Design review of the part shown in the three views and the two pictorial views. Dimensions are in mm from the part's minimum x, y and z. Coordinates: 2 decimals unless noted, no trailing zeros. Loops run counter-clockwise (first coordinate to the right, second up) from the corner with the lowest first, then second, coordinate; pieces in that order, holes last. Notation, with made-up numbers: M 18,13 L 66,13 A30 ccw 66,46 Z; hole C 37.5,-9.5 d10. An arc over 180 degrees is marked long. Use one line per item in the form item = value.
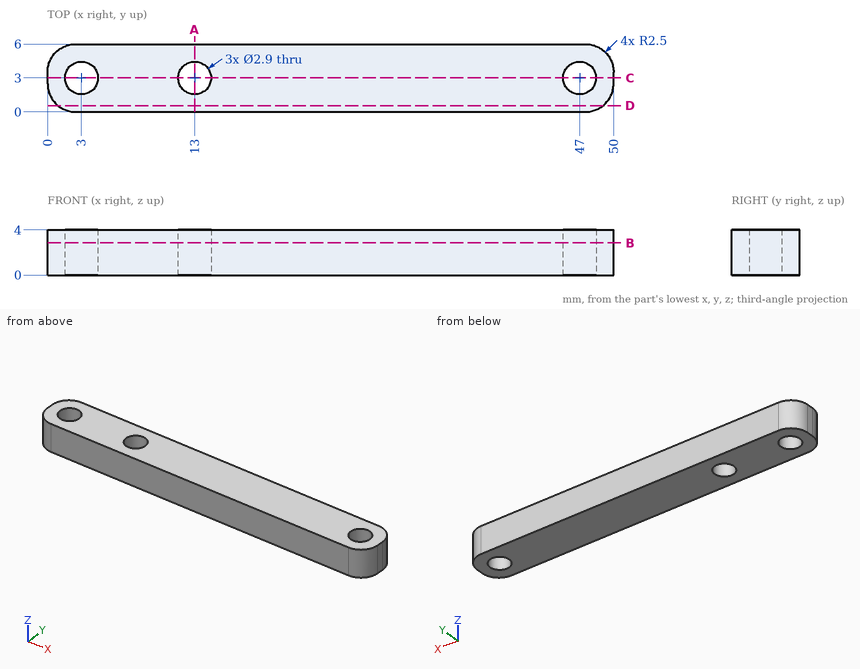
1. Add section D-D (y = 0.55). State the section outline as (x, z) points, then the cut area to 3 significant figures.
Response values:
outline = M 0.94,0 L 49.06,0 L 49.06,4 L 0.94,4 Z
area = 193 mm^2
2. Wall thickness on line 1 along Y through (x, z) = (3, 1.6); line 2 along X through (y, z) = (1.9, 1.3); line 3 along X through (y, z) = (2.2, 2.55): over which ranges is each line inside the solid? List them lowest first. Write a range as from..to.
Response values:
line_1 = 0..1.55, 4.45..6
line_2 = 0.07..2.06, 3.94..12.06, 13.94..46.06, 47.94..49.93
line_3 = 0.02..1.79, 4.21..11.79, 14.21..45.79, 48.21..49.98
3. Insertion check: P1, Ø1, axis at y = 1, z = 2, coming from the +X side. The pin has a flat end and moves straight along its axis. Give the tip position at first contact, or say it passes through.
Response values:
P1 = 49.79
4. Add section B-B (z = 2.85). State the section outline as (x, y) points, then the cut area to 3 significant figures.
Response values:
outline = M 0,2.5 A2.5 ccw 2.5,0 L 47.5,0 A2.5 ccw 50,2.5 L 50,3.5 A2.5 ccw 47.5,6 L 2.5,6 A2.5 ccw 0,3.5 Z; hole C 3,3 d2.9; hole C 13,3 d2.9; hole C 47,3 d2.9
area = 275 mm^2
5. Add section C-C (y = 3). State the section outline as (x, z) points.
Response values:
outline = M 0,0 L 1.55,0 L 1.55,4 L 0,4 Z; M 4.45,0 L 11.55,0 L 11.55,4 L 4.45,4 Z; M 14.45,0 L 45.55,0 L 45.55,4 L 14.45,4 Z; M 48.45,0 L 50,0 L 50,4 L 48.45,4 Z
6. Add section A-A (x = 13). State the section outline as (y, z) points, then the cut area to 3 significant figures.
Response values:
outline = M 0,0 L 1.55,0 L 1.55,4 L 0,4 Z; M 4.45,0 L 6,0 L 6,4 L 4.45,4 Z
area = 12.4 mm^2
